Input: part model. Units: mm. Frame: model coordinates. Round coordinates to 2 decimals unless told otherwise and drop trailing zeros. Loops run counter-clockwise (first coordinate to the right, second up) from the corner with the lowest first, then second, coordinate; pieces in that order, holes last. Notation, with made-up numbers: (-8.75, 65) - (49.25, 65) arc R18 ccw to (49.25, 96) - close; hole circle Ø10 at (5.25, 25). An arc over 180 degrees is marked (long way). Write each question's results on one line, items separated by ' | '.
Autodesk Inventor part; units mm, degrees
ref_plane "YZ Plane" through (0, 0, 0) normal (1, 0, 0) x (0, 1, 0)
ref_plane "XZ Plane" through (0, 0, 0) normal (0, 1, 0) x (-1, 0, 0)
ref_plane "XY Plane" through (0, 0, 0) normal (0, 0, 1) x (1, 0, 0)
sketch "Sketch1" plane through (0, 0, 0) normal (0, 0, 1) x (1, 0, 0)
  line L0 (-11.1101, 6.0966) -> (-9.5601, 3.3251)
  line L1 (-9.5601, 3.3251) -> (-11.1853, 0.5971)
  line L2 (-11.1853, 0.5971) -> (-14.3604, 0.6405)
  line L3 (-14.3604, 0.6405) -> (-15.9104, 3.412)
  line L4 (-15.9104, 3.412) -> (-14.2852, 6.14)
  line L5 (-14.2852, 6.14) -> (-11.1101, 6.0966)
  circle A0 centre (-12.7353, 3.3685) radius 1.5
  dimension "d0" = 5.5
  dimension "d1" = 3
extrude "Extrusion1" add sketch "Sketch1" along normal blind 8
thread "Thread2"
thread "Thread3"
properties part number "Espaciador para Electrónica 5mm" material "Acetal Resin, White"
1. Section query D-D, the plane x = -10.75. Output: boundary loops of the cut face in (y, z), plus the area to 3 significant figures.
Answer:
outline: (1.33, 0) - (5.45, 0) - (5.45, 8) - (1.33, 8) - close | area: 33.0 mm^2
2. Line query: line 1 (X direction, y = 2.45, z = 5.5); line 2 (Y direction, x = -13.25, z = 4.25); line 3 (X direction, y = 4.7, z = 3). Output: solid intervals per line, ascending. Write a range as [from, to].
Answer:
line 1: [-15.37, -13.92], [-11.55, -10.08] | line 2: [0.63, 1.96], [4.78, 6.13] | line 3: [-15.14, -13.43], [-12.04, -10.33]
3. Section query C-C, the plane z = 5.5. Output: boundary loops of the cut face in (x, y).
Answer:
outline: (-15.91, 3.41) - (-14.36, 0.64) - (-11.19, 0.6) - (-9.56, 3.33) - (-11.11, 6.1) - (-14.29, 6.14) - close; hole circle Ø3 at (-12.74, 3.37)
4. Section query B-B, the plane y = 3.9. Output: boundary loops of the cut face in (x, z).
Answer:
outline: (-15.62, 0) - (-14.14, 0) - (-14.14, 8) - (-15.62, 8) - close; (-11.33, 0) - (-9.88, 0) - (-9.88, 8) - (-11.33, 8) - close
5. Mould query, pull axis Y, two halves, no side actions, for faces 1 (the flat face through (-11, 4, 8)), 2 (the flat face through (-10.346, 4.73, 3.944)), 3 (the cylindrical face through (-11.35, 3.94, 3.94)). Classes: pulls with the +Y half, pulls with the -Y half, needs draft (parallel to the pull), parting line crosses it, or undercut.
Answer:
face 1: needs draft | face 2: pulls with the +Y half | face 3: undercut
6. Section query A-A, the plane x = -13.75. Output: boundary loops of the cut face in (y, z).
Answer:
outline: (0.63, 0) - (2.26, 0) - (2.26, 8) - (0.63, 8) - close; (4.47, 0) - (6.13, 0) - (6.13, 8) - (4.47, 8) - close
